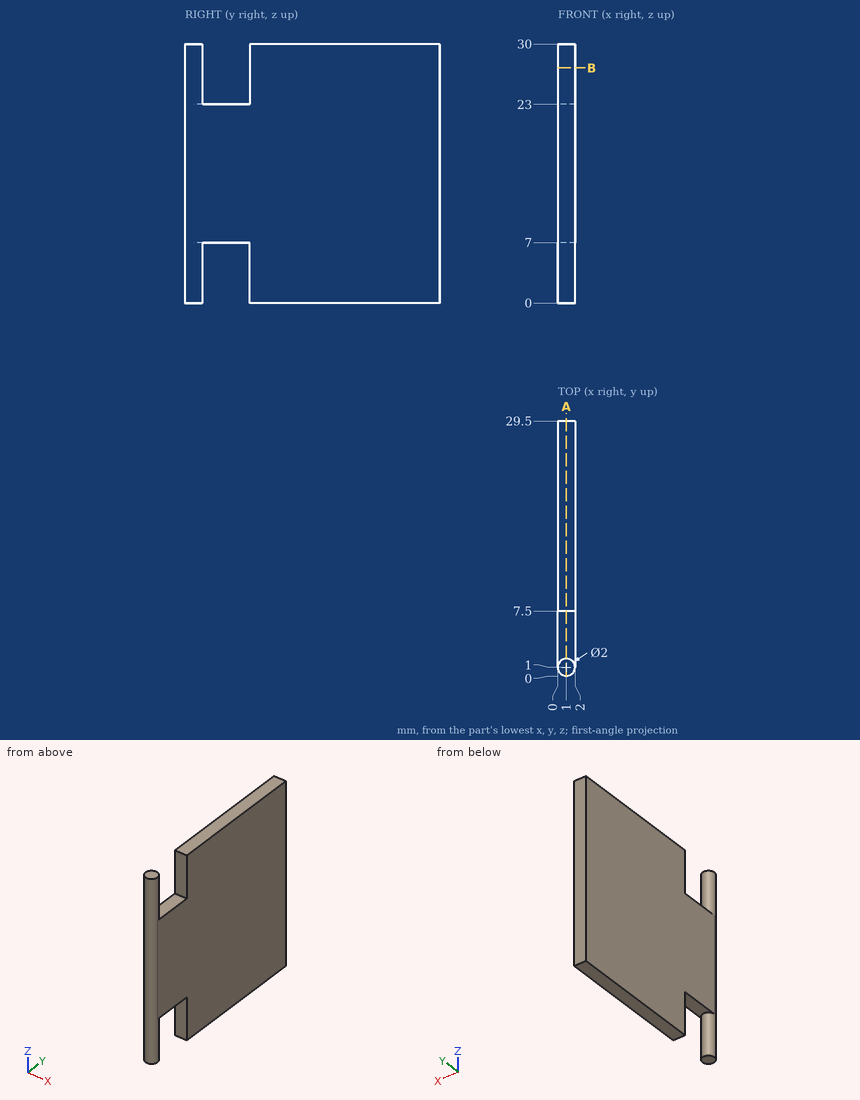
For this review, use the dimensioned drawing (mm, ordinates from the lowest corner) and the shaded views. Coordinates: 2 decimals unless noted, no trailing zeros. Order: outer loops, then holes, each group sorted by start corner. A loop starts at its lowest first (then second) coordinate and runs counter-clockwise, first axis right, second up. Notation, with made-up numbers: (84.5, -26) -> (106.5, -26) arc R15 cw to (106.5, 3) -> close; hole circle Ø11 at (21.5, 61.5). An arc over 180 degrees is marked (long way). One line per item, written item: value. Start each with the question number.
Q1. Insertion check: pin 1 Ø0.6 at (x, y) = (1, 5) entering from +Z; pin 2 Ø1 at (x, y) = (1.5, 5) entering from -Z. Each pin has a flat end and moves straight along its axis. Give the tip position at first contact, or say it passes through.
Q2. Take a section at B-B, the plane z = 27.25. State the section outline as (x, y) points, then the cut area to 3 significant figures.
Q3. Take a section at A-A, the plane x = 1. State the section outline as (y, z) points, then the cut area to 3 significant figures.
Q4. For probe 1 along Y at (x, z) = (0.45, 28.25); probe 2 along Y at (x, z) = (0.85, 19.75); probe 3 along Y at (x, z) = (0.1, 6), list the stretches that pass through material, from the lowest coordinate up.
Values follow:
1. pin 1: stops at z = 23
1. pin 2: stops at z = 7
2. outline: circle Ø2 at (1, 1); (0, 7.5) -> (2, 7.5) -> (2, 29.5) -> (0, 29.5) -> close
2. area: 47.1 mm2
3. outline: (0, 0) -> (2, 0) -> (2, 7) -> (7.5, 7) -> (7.5, 0) -> (29.5, 0) -> (29.5, 30) -> (7.5, 30) -> (7.5, 23) -> (2, 23) -> (2, 30) -> (0, 30) -> close
3. area: 808 mm2
4. probe 1: y = 0.16 to 1.84, 7.5 to 29.5
4. probe 2: y = 0.01 to 29.5
4. probe 3: y = 0.56 to 1.44, 7.5 to 29.5
